Geometry: final body of the model. Coordinates: model frame, mm. A direction names the side the tool comes from. Round coordinates to 2 decimals unless told otherwise and drop trailing zeros. Order: outer loops, then holes, each group sorted by start corner. A loop starts at its lowest first (then second) coordinate and runs counter-clockwise, first axis right, second up. Notation, with made-up numbers: (15, 84.5) -> (63, 84.5) arc R10 cw to (63, 100.5) -> close; hole circle Ø6 at (83, -38.75). An arc over 180 degrees is marked (long way). Put each result on its own line as item: value.
```python
from build123d import *

# Parameters (mm, degrees)
ESBO_O1_R                  = 10
RESSALTO_EXTRUS_O1_DEPTH   = 17
CORTE_EXTRUS_O1_START      = -5
CORTE_EXTRUS_O1_DEPTH      = 5
CORTE_EXTRUS_O2_DEPTH      = 15
CORTE_EXTRUS_O3_REACH      = 25.472
CORTE_EXTRUS_O3_END_RADIUS = 10
ESBO_O4_R                  = 1.5


with BuildPart() as part:
    # Esboço1 → Ressalto-extrusão1 (new body)
    with BuildSketch(Plane.XY):
        Circle(ESBO_O1_R)
    extrude(amount=RESSALTO_EXTRUS_O1_DEPTH)

    # Esboço2 → Corte-extrusão1 (cut)
    with BuildSketch(Plane.XY.offset(17).offset(CORTE_EXTRUS_O1_START)):
        with BuildLine():
            Line((-5, 8.660254038), (-5, -8.660254038))
            ThreePointArc((-5, -8.660254038), (-10, 0), (-5, 8.660254038))
        make_face()
        with BuildLine():
            Line((5, 8.660254038), (5, -8.660254038))
            ThreePointArc((5, -8.660254038), (10, 0), (5, 8.660254038))
        make_face()
    extrude(amount=CORTE_EXTRUS_O1_DEPTH, mode=Mode.SUBTRACT)

    # Esboço3 → Corte-extrusão2 (cut)
    with BuildSketch(Plane(origin=(0, 0, 0), x_dir=(-1, 0, 0), z_dir=(0, 0, -1))):
        with BuildLine():
            Line((0, -2.725), (1.629417074, -2.725))
            ThreePointArc((1.629417074, -2.725), (0, 3.175), (-1.629417074, -2.725))
            Line((-1.629417074, -2.725), (0, -2.725))
        make_face()
    extrude(amount=-CORTE_EXTRUS_O2_DEPTH, mode=Mode.SUBTRACT)

    # Corte-extrusão3: up to this cylinder (the profile starts inside it)
    corte_extrus_o3_end = Plane(origin=(0, 0, 7), z_dir=(0, 0, -1)) * Cylinder(CORTE_EXTRUS_O3_END_RADIUS, 71.944, mode=Mode.PRIVATE)
    # Esboço4 → Corte-extrusão3 (cut, up to the surface)
    with BuildSketch(Plane(origin=(0, -2.725, 0), x_dir=(1, 0, 0), z_dir=(0, 1, 0)), mode=Mode.PRIVATE) as corte_extrus_o3_sk1:
        with Locations(Location((0, -7, 0), (0, 0, 270))):
            Circle(ESBO_O4_R)
    corte_extrus_o3_tool1 = extrude(corte_extrus_o3_sk1.sketch, amount=-CORTE_EXTRUS_O3_REACH, mode=Mode.PRIVATE) & corte_extrus_o3_end
    add(corte_extrus_o3_tool1.solids().sort_by_distance((0, -2.725, 7))[0], mode=Mode.SUBTRACT)


solid = part.part
```
1. Cut plane C-C on z = 12.5. Return loops of the section in (x, y) (3 decimals), and give its area (3 significant figures).
Ans:
outline: (-5, -8.66) arc R10 ccw to (5, -8.66) -> (5, 8.66) arc R10 ccw to (-5, 8.66) -> close; hole (-1.629, -2.725) -> (1.629, -2.725) arc R3.175 ccw (long way) to start
area: 161 mm²
2. Draft query along X for faces 1 (the face through (0, 0, 15)), 2 (the face through (-5, 0, 14)), 3 (the face through (7, 0, 12)). Return one class per face: +X half, -X half, draft (parallel to the pull), parting line (faces both ways), or undercut.
Ans:
face 1: undercut
face 2: -X half
face 3: draft
3. Cut plane A-A on x = 0. Return loops of the section in (y, z) (3 decimals).
Ans:
outline: (-10, 0) -> (-2.725, 0) -> (-2.725, 5.5) -> (-10, 5.5) -> close; (-10, 8.5) -> (-2.725, 8.5) -> (-2.725, 15) -> (3.175, 15) -> (3.175, 0) -> (10, 0) -> (10, 17) -> (-10, 17) -> close
4. Set-up query: faces 4 (the face through (-7, 0, 12)), 5 (the face through (0, -2.725, 9)), 6 (the face through (5, 0, 14)). Return all of +Z, -Z, +X, -X, +Y, -Y with unobstructed straight access to the full face (end or side cutting, diameter ignored); none if empty.
Ans:
face 4: +Z, -X, +Y, -Y
face 5: -Z
face 6: +Z, +X, +Y, -Y
5. Cut plane D-D on z = 7. Return loops of the section in (x, y) (3 decimals).
Ans:
outline: (-1.629, -2.725) arc R3.175 cw (long way) to (1.629, -2.725) -> (1.5, -2.725) -> (1.5, -9.887) arc R10 ccw (long way) to (-1.5, -9.887) -> (-1.5, -2.725) -> close
6. Contact query for flat-ended pins moving along their axis: P1, Ø2.5, axis at y = -2.5, z = 15, coming from the -X side; P2, Ø2.5, axis at x = 0, z = 7, coming from the -Y side; P3, Ø1.5, axis at y = 1.5, z = 15, coming from the +X side. Output: stop coordinate, or through.
Ans:
P1: x = -5
P2: y = 2.92
P3: x = 5
7. Cut plane B-B on y = 0. Return loops of the section in (x, z) (3 decimals).
Ans:
outline: (-10, 0) -> (-3.175, 0) -> (-3.175, 15) -> (3.175, 15) -> (3.175, 0) -> (10, 0) -> (10, 12) -> (5, 12) -> (5, 17) -> (-5, 17) -> (-5, 12) -> (-10, 12) -> close
8. Material intervals for probe 1 along Z at (x, y) = (0, -5.5); probe 2 along X at (y, z) = (-8, 7); probe 3 along X at (y, z) = (-6.75, 13.25), sorted ascending.
Ans:
probe 1: 0 to 5.5, 8.5 to 17
probe 2: -6 to -1.5, 1.5 to 6
probe 3: -5 to 5
